Design review of the part built by this model. Coordinates are the model's own, in mm. Face numbers are marked on the shaded views. A direction names the side the tool comes from. Coordinates: 2 decimals unless noted, no trailing zeros. Write each loop counter-clockwise with the first axis right and the second up, starting at its lowest first coordinate (ties: lowest second). Pieces come first, ordered by that corner, then holes. Notation, with made-up numbers: (-31, 16.5) -> (-15, 16.5) arc R20 cw to (-15, 24.5) -> close; hole circle Ø3 at (12.5, 63.5). An arc over 180 degrees is marked (long way). One line per question, with ' | ' between items. Start each with the question number.
Q1. For the marked faces 1 and 2, list the 3-axis set-ups (+Z, -Z, +X, -X, +Y, -Y) from which the entire face can be reached by the end or side of a thin tool; tool diameter is ignored.
Q2. Wall thickness on probe 1 along X at (y, z) = (-8, 3.5); probe 2 along Z at (x, y) = (13.5, -0.25); probe 3 along Y at (x, z) = (31.5, 3): over which ranges is each line inside the solid? List them lowest first.
Q3. Add section A-A on x = 56.5. State the section outline as (y, z) points.
Q4. For P1, Ø6, axis at y = 3, z = -1, coming from the -X side; P2, Ø1, axis at x = 57.5, z = -7, coming from the +Y side; P3, Ø1.5, axis at x = 15.5, z = -4.5, coming from the +Y side; P4, Ø4, axis at x = 58, z = -4, coming from the -Y side, all flat-tipped, find the tip position at first contact; note any pin that passes through.
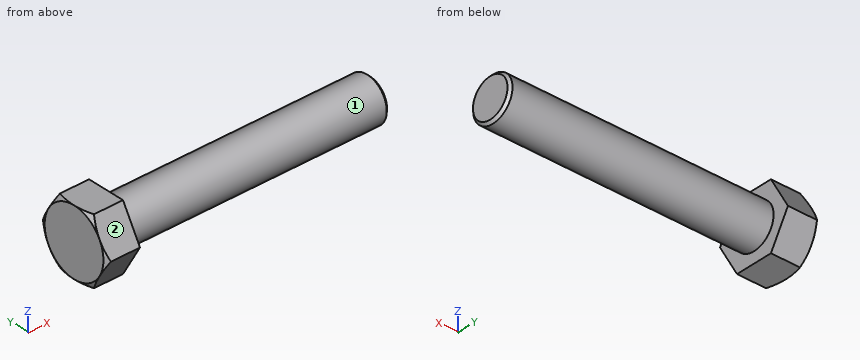
from build123d import *

# Parameters (mm, degrees)
BASEHEAD_DEPTH = 9.2456


with BuildPart() as part:
    # Sketch1 → BaseHead (new body)
    with BuildSketch(Plane(origin=(0, 0, 0), x_dir=(0, 0, -1), z_dir=(1, 0, 0))):
        Polygon((9.525, 5.499261314), (9.525, -5.499261314), (0, -10.998522628), (-9.525, -5.499261314), (-9.525, 5.499261314), (0, 10.998522628), align=None)
    extrude(amount=BASEHEAD_DEPTH)

    # BodySke → BaseBody (revolve)
    with BuildSketch(Plane.XY):
        Polygon((0, 0), (85.4456, 0), (85.4456, 5.59435), (84.68995, 6.35), (0, 6.35), align=None)
    revolve(axis=Axis((0, 0, 0), (1, 0, 0)))

    # Sketch3 → HeadChamfer (revolve, cut)
    with BuildSketch(Plane.XY):
        Polygon((0, 9.525), (4.516912895, 17.348522628), (4.516912895, 23.698522628), (-12.7, 23.698522628), (-12.7, 9.525), align=None)
    revolve(axis=Axis((0, 0, 0), (1, 0, 0)), mode=Mode.SUBTRACT)


solid = part.part
Output values:
1) face 1: +X | face 2: +Z, +X, -X, -Y
2) probe 1: x = 0 to 9.25 | probe 2: z = -6.35 to 6.35 | probe 3: y = -5.6 to 5.6
3) outline: circle Ø12.7 at (0, 0)
4) P1: stops at x = 0 | P2: passes through | P3: stops at y = 5.12 | P4: stops at y = -6.03
